Could you check a few things on this drawing? It's one solid part, dimensions in mm from its lowest x, y, z. A direction names the side the tool comes from. Give positions to 0.01 mm unless a question says otherwise; leave off trailing zeros. Order: outer loops, then holes, each group sorted by start corner. A loop starts at its lowest first (then second) coordinate and runs counter-clockwise, first axis right, second up. Notation, with made-up numbers: M -10,-15 L -3,-15 A31 ccw -3,20 Z; hole C 61,42 d9. An arc over 180 degrees is marked long. Use one line per item in the form item = value.
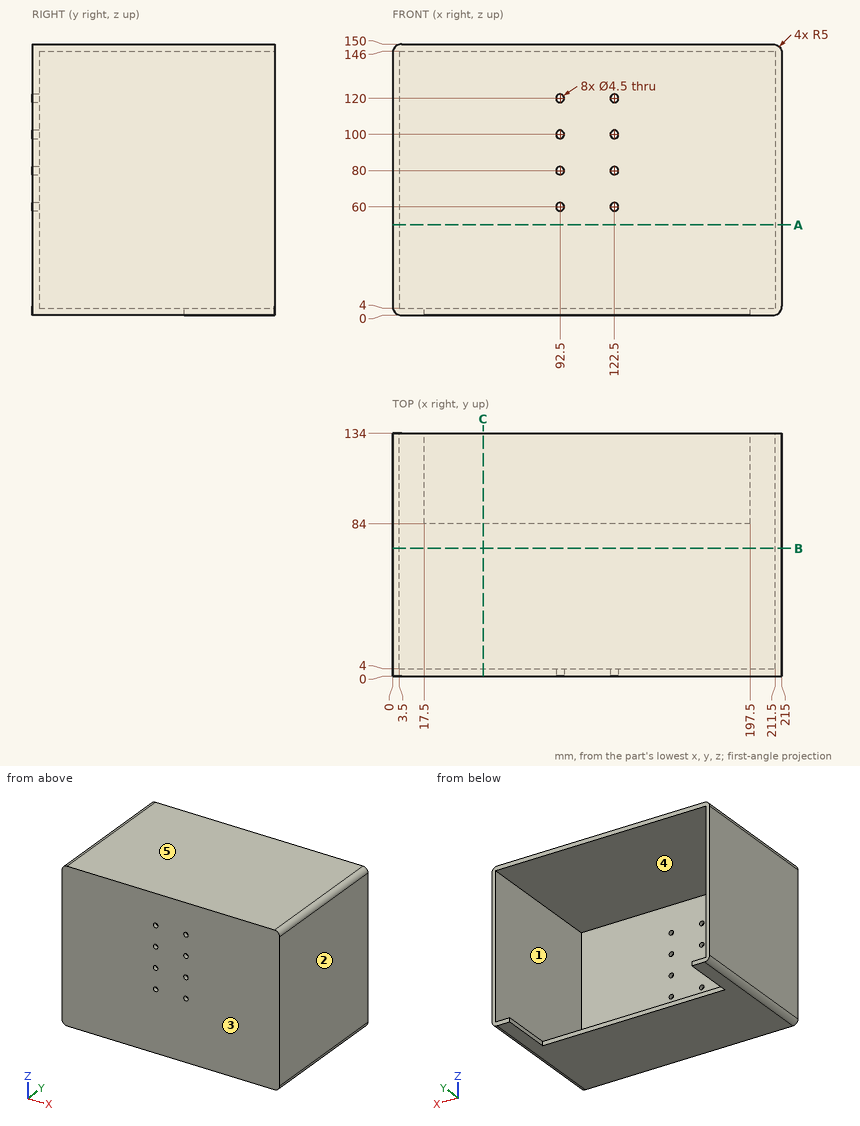
Q1. I want a section at A-A on z = 50. Write out the boundary of the cut face in (x, y).
Found:
outline = M 0,0 L 215,0 L 215,134 L 211.5,134 L 211.5,4 L 3.5,4 L 3.5,134 L 0,134 Z
Q2. On a 3-axis mill with a long thin cutter (end or side, diameter ignored), from which of +Z, -Z, +X, -X, +Y, -Y can I reach the whole of each face in a straight line? I mean the marked faces 4 and 5. Say none if no direction works.
Found:
face_4 = +Y
face_5 = +Z, +X, -X, +Y, -Y
Q3. I'm going to push flat-ended pins straight in: pin 1 Ø1.2 at (y, z) = (97.5, 2.5) entering from +X; pin 2 Ø5 at (x, z) = (94, 47.5) entering from -Y; pin 3 Ø3.5 at (x, z) = (92.5, 120) entering from -Y; pin 4 Ø1.5 at (x, z) = (193, 106.5) entering from +Y. Where does each tip first touch, or does it pass through?
Found:
pin_1 = 214.62
pin_2 = 0
pin_3 = through
pin_4 = 4
Q4. I need wall thicknesses on L1, parallel to Z at x = 122, y = 1; L2, parallel to X at y = 1.3, z = 120; L3, parallel to X at y = 34.5, z = 118. Which ranges of each line are inside material? Lowest first, please.
Found:
L1 = 0 to 57.81, 62.19 to 77.81, 82.19 to 97.81, 102.19 to 117.81, 122.19 to 150
L2 = 0 to 90.25, 94.75 to 120.25, 124.75 to 215
L3 = 0 to 3.5, 211.5 to 215
Q5. I want a section at C-C on x = 50. Write out the boundary of the cut face in (y, z).
Found:
outline = M 0,0 L 84,0 L 84,4 L 4,4 L 4,146 L 134,146 L 134,150 L 0,150 Z
Q6. I want a section at B-B on y = 70.5. Write out the boundary of the cut face in (x, z).
Found:
outline = M 0,5 A5 ccw 5,0 L 210,0 A5 ccw 215,5 L 215,145 A5 ccw 210,150 L 5,150 A5 ccw 0,145 Z; hole M 3.5,4 L 211.5,4 L 211.5,146 L 3.5,146 Z
Q7. Thinking about a two-plate mould opening in X: for the marked faces 1, 2 and 3, which applies, +X half, -X half, draft (parallel to the pull), parting line (faces both ways), or undercut?
Found:
face_1 = undercut
face_2 = +X half
face_3 = draft
